from build123d import *

# Parameters (mm, degrees)
SKETCH1_R                             = 37.5
BASE_PLATE_DEPTH                      = 5
SKETCH2_R                             = 6
PIN_DEPTH                             = 30
SKETCH11_R                            = 4
SCREWINSERTS_DEPTH                    = 5
INSERTSCIRPATTERN3_COUNT              = 6
SKETCH10_R                            = 2.15
SCREW_HOLES_DEPTH                     = 35
SCREWHOLEPATTERN1_OUTLINE_R           = 2.15
SCREWHOLEPATTERN1_DEPTH               = 5
SKETCH9_R                             = 3.5
PINHOLES_DEPTH                        = 0.5
PINHOLECIRPATTERN2_COUNT              = 6
SKETCH3_R                             = 17.45
OUTPUT_SHAFT_DEPTH                    = 15
SKETCH5_R                             = 16.35
BEARINGHOLE_DEPTH                     = 8
SKETCH6_R                             = 10.65
INPUTSHAFT_HOLE_DEPTH                 = 66.24185773
COMPLIANCE_CUT_DEPTH                  = 8
CHAMFER_2_SIZE                        = 1
WALL_COMPLIANCE_CIT_REACH             = 65.541
SKETCH13_W                            = 1
SKETCH13_H                            = 31.47761194
WALL_COMPLIANCE_CIT_DIRECTION_2_REACH = 65.541


# Read off the part's stored shape, not the designer's step: ScrewHolePattern1
with BuildPart() as part:
    # Sketch1 → Base Plate (new, symmetric)
    with BuildSketch(Plane.XY):
        Circle(SKETCH1_R)
    extrude(amount=BASE_PLATE_DEPTH, both=True)

    # Sketch11 → ScrewInserts (cut)
    with BuildSketch(Plane(origin=(0, 0, -5), x_dir=(-1, 0, 0), z_dir=(0, 0, -1))):
        with Locations((28, 0)):
            Circle(SKETCH11_R)
    screwinserts = extrude(amount=-SCREWINSERTS_DEPTH, mode=Mode.SUBTRACT)

    # InsertsCirPattern3: ScrewInserts ×6 about axis
    insertscirpattern3_axis = Axis((0, 0, 0), (0, 0, 1))
    for i in range(1, INSERTSCIRPATTERN3_COUNT):
        add(screwinserts.rotate(insertscirpattern3_axis, i * 360 / INSERTSCIRPATTERN3_COUNT), mode=Mode.SUBTRACT)


with BuildPart() as body_2:
    # Sketch2 → Pin (new body)
    with BuildSketch(Plane.XY.offset(5)):
        with Locations((-28, 0)):
            Circle(SKETCH2_R)
    extrude(amount=PIN_DEPTH)


with BuildPart() as screw_holes_tool:
    # Sketch10 → Screw Holes (new body)
    with BuildSketch(Plane.XY.offset(35)):
        with Locations((-28, 0)):
            Circle(SKETCH10_R)
    extrude(amount=-SCREW_HOLES_DEPTH)


with BuildPart() as part_1:
    add(part.part)

    # Screw Holes: cut by screw_holes_tool
    add(screw_holes_tool.part, mode=Mode.SUBTRACT)

    # ScrewHolePattern1 outline → ScrewHolePattern1 (cut)
    with BuildSketch(Plane.XY):
        with Locations((-14, 24.248711306)):
            Circle(SCREWHOLEPATTERN1_OUTLINE_R)
        with Locations((14, 24.248711306)):
            Circle(SCREWHOLEPATTERN1_OUTLINE_R)
        with Locations((28, 0)):
            Circle(SCREWHOLEPATTERN1_OUTLINE_R)
        with Locations((14, -24.248711306)):
            Circle(SCREWHOLEPATTERN1_OUTLINE_R)
        with Locations((-14, -24.248711306)):
            Circle(SCREWHOLEPATTERN1_OUTLINE_R)
    extrude(amount=SCREWHOLEPATTERN1_DEPTH, mode=Mode.SUBTRACT)

    # Sketch9 → PinHoles (cut)
    with BuildSketch(Plane.XY.offset(5)):
        with Locations((-28, 0)):
            Circle(SKETCH9_R)
    pinholes = extrude(amount=-PINHOLES_DEPTH, mode=Mode.SUBTRACT)

    # PinHoleCirPattern2: PinHoles ×6 about axis
    pinholecirpattern2_axis = Axis((0, 0, 0), (0, 0, 1))
    for i in range(1, PINHOLECIRPATTERN2_COUNT):
        add(pinholes.rotate(pinholecirpattern2_axis, i * 360 / PINHOLECIRPATTERN2_COUNT), mode=Mode.SUBTRACT)

    # Sketch3 → Output Shaft (add)
    with BuildSketch(Plane(origin=(0, 0, -5), x_dir=(-1, 0, 0), z_dir=(0, 0, -1))):
        Circle(SKETCH3_R)
    extrude(amount=OUTPUT_SHAFT_DEPTH)

    # Sketch5 → BearingHole (cut)
    with BuildSketch(Plane.XY.offset(5)):
        Circle(SKETCH5_R)
    extrude(amount=-BEARINGHOLE_DEPTH, mode=Mode.SUBTRACT)

    # Sketch6 → InputShaft Hole (cut, through all)
    with BuildSketch(Plane.XY.offset(-3)):
        Circle(SKETCH6_R)
    extrude(amount=-INPUTSHAFT_HOLE_DEPTH, mode=Mode.SUBTRACT)

    # Sketch12 → Compliance Cut (cut)
    with BuildSketch(Plane.XY.offset(5)):
        with BuildLine():
            Line((-7.858753082, 18.5), (-6.685804861, 15.73880597))
            ThreePointArc((-6.685804861, 15.73880597), (-17.1, 0), (-6.685804861, -15.73880597))
            Line((-6.685804861, -15.73880597), (-7.858753082, -18.5))
            ThreePointArc((-7.858753082, -18.5), (-20.1, 0), (-7.858753082, 18.5))
        make_face()
    compliance_cut = extrude(amount=-COMPLIANCE_CUT_DEPTH, mode=Mode.SUBTRACT)

    # Mirror1: Compliance Cut across plane
    add(compliance_cut.mirror(Plane(origin=(0, 0, 0), x_dir=(0, 0, 1), z_dir=(1, 0, 0))), mode=Mode.SUBTRACT)

    # Chamfer 2
    # the kernel refuses this chamfer: 1 mm, written as the material it takes off along each edge
    with BuildSketch(Plane(origin=(0, 0, 5), x_dir=(1, 0, 0), z_dir=(0, -1, 0))) as chamfer_2_piece_1:
        Polygon((37.5, -CHAMFER_2_SIZE), (37.5 - CHAMFER_2_SIZE, 0), (37.5, 0), align=None)
    revolve(axis=Axis((0, 0, 5), (0, 0, 1)), mode=Mode.SUBTRACT)
    with BuildSketch(Plane(origin=(0, 0, -5), x_dir=(1, 0, 0), z_dir=(0, -1, 0))) as chamfer_2_piece_2:
        Polygon((37.5, CHAMFER_2_SIZE), (37.5 - CHAMFER_2_SIZE, 0), (37.5, 0), align=None)
    revolve(axis=Axis((0, 0, -5), (0, 0, 1)), mode=Mode.SUBTRACT)
    with BuildSketch(Plane(origin=(0, 0, -20), x_dir=(1, 0, 0), z_dir=(0, -1, 0))) as chamfer_2_piece_3:
        Polygon((10.65 + CHAMFER_2_SIZE, 0), (10.65, CHAMFER_2_SIZE), (10.65, 0), align=None)
    revolve(axis=Axis((0, 0, -20), (0, 0, 1)), mode=Mode.SUBTRACT)
    with BuildSketch(Plane(origin=(0, 0, -3), x_dir=(1, 0, 0), z_dir=(0, -1, 0))) as chamfer_2_piece_4:
        Polygon((10.65 + CHAMFER_2_SIZE, 0), (10.65, -CHAMFER_2_SIZE), (10.65, 0), align=None)
    revolve(axis=Axis((0, 0, -3), (0, 0, 1)), mode=Mode.SUBTRACT)
    with BuildSketch(Plane(origin=(0, 0, 5), x_dir=(1, 0, 0), z_dir=(0, -1, 0))) as chamfer_2_piece_5:
        Polygon((16.35 + CHAMFER_2_SIZE, 0), (16.35, -CHAMFER_2_SIZE), (16.35, 0), align=None)
    revolve(axis=Axis((0, 0, 5), (0, 0, 1)), mode=Mode.SUBTRACT)

    # Sketch13 → Wall Compliance Cit (cut, up to next)
    with BuildSketch(Plane(origin=(0, 0, 0), x_dir=(0, 0, -1), z_dir=(1, 0, 0)), mode=Mode.PRIVATE) as wall_compliance_cit_sk1:
        with Locations((2.5, 0)):
            Rectangle(SKETCH13_W, SKETCH13_H)
    wall_compliance_cit_tool1 = extrude(wall_compliance_cit_sk1.sketch, amount=-WALL_COMPLIANCE_CIT_REACH, mode=Mode.PRIVATE) & part_1.part
    add(wall_compliance_cit_tool1.solids().sort_by_distance((0, 0, -2.5))[0], mode=Mode.SUBTRACT)

    # Sketch13 → Wall Compliance Cit direction 2 (cut, up to next)
    with BuildSketch(Plane(origin=(0, 0, 0), x_dir=(0, 0, -1), z_dir=(1, 0, 0)), mode=Mode.PRIVATE) as wall_compliance_cit_direction_2_sk1:
        with Locations((2.5, 0)):
            Rectangle(SKETCH13_W, SKETCH13_H)
    wall_compliance_cit_direction_2_tool1 = extrude(wall_compliance_cit_direction_2_sk1.sketch, amount=WALL_COMPLIANCE_CIT_DIRECTION_2_REACH, mode=Mode.PRIVATE) & part_1.part
    add(wall_compliance_cit_direction_2_tool1.solids().sort_by_distance((0, 0, -2.5))[0], mode=Mode.SUBTRACT)


with BuildPart() as body_2_1:
    add(body_2.part)

    # Screw Holes: cut by screw_holes_tool
    add(screw_holes_tool.part, mode=Mode.SUBTRACT)


solid = part_1.part
Design review of the part built by this model. Coordinates are the model's own, in mm. A direction names the side the tool comes from. Round coordinates to 2 decimals unless told otherwise and drop trailing zeros. Write each loop counter-clockwise with the first axis right and the second up, starting at its lowest first coordinate (ties: lowest second). Pieces come first, ordered by that corner, then holes. Notation, with made-up numbers: (22, 70.5) -> (44, 70.5) arc R25 ccw to (44, 85.5) -> close; hole circle Ø4 at (34.5, 25.5). An arc over 180 degrees is marked (long way). One line per question, with ' | ' between items.
(1) Take a section at A-A, the plane y = 0. State how many separate pieces and enclosed holes the cut face has, and give its area (3 significant figures).
Result sheet:
separate pieces: 6 | enclosed holes: 0 | area: 470 mm2
(2) Take a section at B-B, the plane z = -17.25. State the section outline as (x, y) points.
Result sheet:
outline: circle Ø34.9 at (0, 0); hole circle Ø21.3 at (0, 0)
(3) Machinability: for faces 1 (the cylindrical face through (-17.098, 0.28, 1.422)), 2 (the cylindrical face through (24.8, 2.4, -2.5)), 3 (the cylindrical face through (-30.15, 0.09, 2.28)), which of the approach directions +Z, -Z, +X, -X, +Y, -Y give a long, thin tool a straight path to every point of the face, cutting with its end or side? Answer none if there is none.
Result sheet:
face 1: +Z | face 2: -Z | face 3: +Z, -Z
(4) Draft analysis for pull direction Z (two halves, no side actions). For faces 4 (the flat face through (30, 2, 0)), 5 (the flat face through (16.8, -0.1, -2)), 6 (the flat face through (15, 22, 4.5)), 7 (the cylindrical face through (24.66, -1.05, 4.75)), state which applies: released by +Z, released by -Z, zero draft, split by the parting line, or undercut.
Result sheet:
face 4: released by -Z | face 5: undercut | face 6: released by +Z | face 7: zero draft
(5) Insertion check: P1, Ø6, axis at y = -22.5, z = -1, coming from the -X side; P2, Ø1.1, axis at x = 6, z = -2.5, coming from the -Y side; P3, Ø2, axis at x = -28, y = 1.5, coming from the +Z side. Each pin has a flat end and moves straight along its axis. Give the tip position at first contact, or say it passes through.
Result sheet:
P1: x = -32.03 | P2: y = -37.1 | P3: z = 4.5
(6) Wall thickness on line 1 (Y direction, x = -14, z = -0.25); line 2 (Z direction, x = -18, y = -11.5); line 3 (Y direction, x = -28, z = -1.9): over which ranges is each line inside the solid? List them lowest first. Write a range as [from, to].
Result sheet:
line 1: [-34.79, -28.25], [-20.25, -14.42], [-9.82, -8.45], [8.45, 9.82], [14.42, 20.25], [28.25, 34.79] | line 2: [-5, 5] | line 3: [-24.94, -4], [4, 24.94]
